Part model, mm, in its own coordinate system. A direction names the side the tool comes from. Coordinates: 2 decimals unless noted, no trailing zeros. Write each loop counter-clockwise with the first axis right and the second up, starting at its lowest first coordinate (ties: lowest second). Pieces come first, ordered by that corner, then holes. Notation, with made-up numbers: (-28.5, 81.25) -> (-21.5, 81.25) arc R21 cw to (-21.5, 112.25) -> close; hole circle Ø11 at (-16, 88.5). An arc over 180 degrees is marked (long way). Write item = value, one per line. Start each with the question number.
Q1. Probe line 1 (Y direction, x = 9, z = -36.5); line 2 (Z direction, x = 8.5, y = 4); line 3 (X direction, y = 5.75, z = -5). List the from-to ranges inside material, lowest first.
Q2. Band-saw the part on D-D, the plane x = 63. List the corners of the cut face in (y, z).
Q3. Pin check, flat tips, straight feed: P1, Ø1, axis at y = 18, z = 50, coming from the -X side; P2, Ø2.5, axis at y = 26, z = 74, coming from the +X side; P3, Ø10, axis at x = -24.5, y = 18, coming from the -Z side. Stop position of each tip, or through.
Q4. Pull direction X, two halves, no side cores. Call faces 4 (the cylindrical face through (-61.075, 14.79, 38.666)), 5 (the flat face through (-11, 20, 20)), 6 (the flat face through (52.45, 30, -43.63)): released by +X, released by -X, zero draft, split by the parting line, or undercut.
Q5. Tool access for faces 1 (the flat face through (14.002, 25, 75)), 2 (the flat face through (74, 25, 14.818)), 3 (the cylindrical face through (-44.76, 24.93, 52.72)): list every direction of +Z, -Z, +X, -X, +Y, -Y with a clear straight run to the whole face (end or side of a thin tool).
Q6. Band-saw the part on B-B, the plane x = -11. List the corners of the cut face in (y, z), plus the area to 3 significant figures.
Q7. Band-saw the part on C-C, the plane z = -20. List the corners of the cut face in (x, y), plus the area to 3 significant figures.
Q8. Band-saw the part on A-A, the plane z = 16.5. List the corners of the cut face in (x, y).
from build123d import *

# Parameters (mm, degrees)
SKETCH1_R                = 68.354
SKETCH1_R_2              = 17.5
BOSS_EXTRUDE2_DEPTH      = 20
BOSS_EXTRUDE3_DEPTH      = 10
BOSS_EXTRUDE3_DEPTH_BACK = 20
SKETCH2_R                = 73.354
SKETCH2_R_2              = 68.354
CUT_EXTRUDE1_DEPTH       = 114.995028009
CUT_EXTRUDE1_DEPTH_BACK  = 114.995028009
CUT_EXTRUDE2_DEPTH       = 114.995028009
CUT_EXTRUDE2_DEPTH_BACK  = 114.995028009


with BuildPart() as part:
    # Sketch1 → Boss-Extrude2 (new body)
    with BuildSketch(Plane(origin=(0, 0, 0), x_dir=(1, 0, 0), z_dir=(0, 1, 0))):
        with Locations(Location((4.002282363, -4.818066557, 0), (0, 0, 270))):
            Circle(SKETCH1_R)
        with Locations(Location((4.002282363, -4.818066557, 0), (0, 0, 270))):
            Circle(SKETCH1_R_2, mode=Mode.SUBTRACT)
    extrude(amount=BOSS_EXTRUDE2_DEPTH)

    # Sketch2 → Boss-Extrude3 (add, two sides: drawn at the far end of the back side and taken through both)
    with BuildSketch(Plane(origin=(0, 20, 0), x_dir=(1, 0, 0), z_dir=(0, 1, 0)).offset(-BOSS_EXTRUDE3_DEPTH_BACK)):
        with Locations(Location((4.002282363, -4.818066557, 0), (0, 0, 270))):
            Circle(SKETCH2_R)
        with Locations(Location((4.002282363, -4.818066557, 0), (0, 0, 270))):
            Circle(SKETCH2_R_2, mode=Mode.SUBTRACT)
    extrude(amount=BOSS_EXTRUDE3_DEPTH + BOSS_EXTRUDE3_DEPTH_BACK)

    # Sketch3 → Cut-Extrude1 (cut, two sides: drawn at the far end of the back side and taken through both)
    with BuildSketch(Plane(origin=(0, 0, 0), x_dir=(0, 0, -1), z_dir=(1, 0, 0)).offset(-CUT_EXTRUDE1_DEPTH_BACK)):
        Polygon((-4.818066557, 30), (5.181933443, 30), (5.181933443, 20), (-14.818066557, 20), (-14.818066557, 30), align=None)
    extrude(amount=CUT_EXTRUDE1_DEPTH + CUT_EXTRUDE1_DEPTH_BACK, mode=Mode.SUBTRACT)

    # Sketch5 → Cut-Extrude2 (cut, two sides: drawn at the far end of the back side and taken through both)
    with BuildSketch(Plane.XY.offset(-CUT_EXTRUDE2_DEPTH_BACK)):
        Polygon((4.002282363, 30), (14.002282363, 30), (14.002282363, 20), (-5.997717637, 20), (-5.997717637, 30), align=None)
    extrude(amount=CUT_EXTRUDE2_DEPTH + CUT_EXTRUDE2_DEPTH_BACK, mode=Mode.SUBTRACT)


solid = part.part
Ans:
q1.line_1 = 0 to 20
q1.line_2 = -68.4 to -12.09, 21.73 to 78.03
q1.line_3 = -68.69 to -10.48, 18.49 to 76.7
q2.outline = (0, -38.77) -> (30, -38.77) -> (30, -29.7) -> (20, -29.7) -> (20, 39.34) -> (30, 39.34) -> (30, 48.41) -> (0, 48.41) -> close
q3.P1 = -54.17
q3.P2 = 31.68
q3.P3 = -64.67
q4.face_4 = split by the parting line
q4.face_5 = undercut
q4.face_6 = zero draft
q5.face_1 = +Z, -Z, +Y
q5.face_2 = +X, -X, +Y
q5.face_3 = +Y
q6.outline = (0, -66.99) -> (30, -66.99) -> (30, -61.87) -> (20, -61.87) -> (20, -4.19) -> (0, -4.19) -> close; (0, 13.83) -> (20, 13.83) -> (20, 71.51) -> (30, 71.51) -> (30, 76.62) -> (0, 76.62) -> close
q6.area = 2,610 mm2
q7.outline = (-65.03, 0) -> (73.03, 0) -> (73.03, 30) -> (67.69, 30) -> (67.69, 20) -> (-59.69, 20) -> (-59.69, 30) -> (-65.03, 30) -> close
q7.area = 2,870 mm2
q8.outline = (-68.42, 0) -> (-9.03, 0) -> (-9.03, 20) -> (-63.35, 20) -> (-63.35, 30) -> (-68.42, 30) -> close; (17.03, 0) -> (76.42, 0) -> (76.42, 30) -> (71.35, 30) -> (71.35, 20) -> (17.03, 20) -> close
